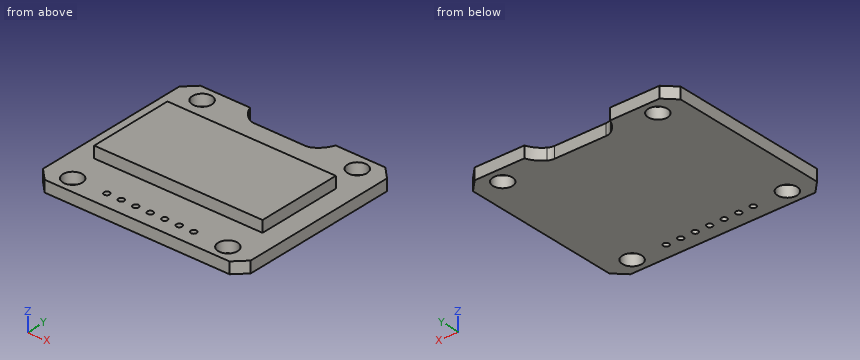
```python
from build123d import *

# Parameters (mm, degrees)
SKETCH_1_W          = 36.4
SKETCH_1_H          = 31.9
EXTRUDE_1_DEPTH     = 2
SKETCH_2_W          = 29.5
SKETCH_2_H          = 15
EXTRUDE_2_DEPTH     = 2
SKETCH_3_R          = 1.7
CUT_EXTRUDE_2_DEPTH = 2
CUT_EXTRUDE_3_DEPTH = 2
SKETCH_5_R          = 0.5
CUT_EXTRUDE_4_DEPTH = 30
CUT_EXTRUDE_5_DEPTH = 10
FILLET_1_R          = 2


with BuildPart() as part:
    # 草图1 → 凸台-拉伸1 (new body)
    with BuildSketch(Plane.XY):
        Rectangle(SKETCH_1_W, SKETCH_1_H)
    extrude(amount=EXTRUDE_1_DEPTH)

    # 草图2 → 凸台-拉伸2 (add)
    with BuildSketch(Plane.XY.offset(2)):
        Rectangle(SKETCH_2_W, SKETCH_2_H)
    extrude(amount=EXTRUDE_2_DEPTH)

    # 草图3 → 切除-拉伸2 (cut)
    with BuildSketch(Plane.XY.offset(2)):
        with Locations((-13.6, 13.25)):
            Circle(SKETCH_3_R)
        with Locations(Location((13.6, 13.25, 0), (0, 0, 180))):
            Circle(SKETCH_3_R)
        with Locations((13.6, -13.25)):
            Circle(SKETCH_3_R)
        with Locations(Location((-13.6, -13.25, 0), (0, 0, 180))):
            Circle(SKETCH_3_R)
    extrude(amount=-CUT_EXTRUDE_2_DEPTH, mode=Mode.SUBTRACT)

    # 草图4 → 切除-拉伸3 (cut)
    with BuildSketch(Plane.XY.offset(2)):
        Polygon((-16.2, 15.95), (-18.2, 13.95), (-18.2, 15.95), align=None)
        Polygon((18.2, 13.95), (18.2, 15.95), (16.2, 15.95), align=None)
        Polygon((16.2, -15.95), (18.2, -13.95), (18.2, -15.95), align=None)
        Polygon((-18.2, -13.95), (-18.2, -15.95), (-16.2, -15.95), align=None)
    extrude(amount=-CUT_EXTRUDE_3_DEPTH, mode=Mode.SUBTRACT)

    # 草图5 → 切除-拉伸4 (cut)
    with BuildSketch(Plane.XY.offset(2)):
        with Locations((-7.62, -13.25)):
            Circle(SKETCH_5_R)
        with Locations((-5.08, -13.25)):
            Circle(SKETCH_5_R)
        with Locations((-2.54, -13.25)):
            Circle(SKETCH_5_R)
        with Locations((0, -13.25)):
            Circle(SKETCH_5_R)
        with Locations((2.54, -13.25)):
            Circle(SKETCH_5_R)
        with Locations((5.08, -13.25)):
            Circle(SKETCH_5_R)
        with Locations((7.62, -13.25)):
            Circle(SKETCH_5_R)
    extrude(amount=-CUT_EXTRUDE_4_DEPTH, mode=Mode.SUBTRACT)

    # 草图6 → 切除-拉伸5 (cut)
    with BuildSketch(Plane.XY.offset(2)):
        with BuildLine():
            Line((-5, 13.25), (5, 13.25))
            ThreePointArc((5, 13.25), (6.519232871, 14.350710305), (7.5, 15.95))
            Line((7.5, 15.95), (-7.5, 15.95))
            ThreePointArc((-7.5, 15.95), (-6.519232871, 14.350710305), (-5, 13.25))
        make_face()
    extrude(amount=-CUT_EXTRUDE_5_DEPTH, mode=Mode.SUBTRACT)

    # 圆角1
    fillet_1_edges = [part.edges().sort_by_distance(p)[0] for p in [
        (-5, 13.25, 1),
        (5, 13.25, 1),
    ]]
    fillet(fillet_1_edges, radius=FILLET_1_R)


solid = part.part
```
Read the model definition and answer for the solid it produces. Units are mm, in the model's axes. Give positions to 0.01 mm unless a question says otherwise; leave off trailing zeros. Write each loop counter-clockwise with the first axis right and the second up, starting at its lowest first coordinate (ties: lowest second). Pieces come first, ordered by that corner, then holes. Notation, with made-up numbers: (83, 65) - (141, 65) arc R29 cw to (141, 95) - close; hole circle Ø4 at (6, -8.75). An arc over 180 degrees is marked (long way). Write item = value, one per line. Start each with the question number.
Item 1: Find section B-B (z = 1.35). State how many separate pieces and enclosed holes the cut face has, then the cut area to 3 significant figures.
Item 2: Find section A-A (x = 2.54). Give the vertices of the cut face in (y, z), then the cut area to 3 significant figures.
Item 3: Find the intervals of material crossed by probe 1 along Y at (x, z) = (13.6, 0.9); probe 2 along Y at (x, z) = (0, 0.2); probe 3 along X at (y, z) = (5, 2.1), in increasing order. Write a range as [from, to].
Item 4: Each of these flat-tipped pins is pushed along its axis until it touches: P1, Ø2, axis at x = 0, z = 2.5, coming from the +Y side; P2, Ø3, axis at x = 13.6, y = 13.25, coming from the -Z side; P3, Ø1.6, axis at y = 3, z = 3, coming from the -X side; P4, Ø1, axis at x = 12.5, z = 3.5, coming from the -Y side. Where does it stop, or does it pass through?
Item 5: Find section C-C (x = -13.6). Give the vertices of the cut face in (y, z), then the cut area to 3 significant figures.
Response:
q1.separate_pieces = 1
q1.enclosed_holes = 11
q1.area = 1,080 mm²
q2.outline = (-15.95, 0) - (-13.75, 0) - (-13.75, 2) - (-15.95, 2) - close; (-12.75, 0) - (13.25, 0) - (13.25, 2) - (7.5, 2) - (7.5, 4) - (-7.5, 4) - (-7.5, 2) - (-12.75, 2) - close
q2.area = 86.4 mm²
q3.probe_1 = [-15.95, -14.95], [-11.55, 11.55], [14.95, 15.95]
q3.probe_2 = [-15.95, -13.75], [-12.75, 13.25]
q3.probe_3 = [-14.75, 14.75]
q4.P1 = 13.25
q4.P2 = through
q4.P3 = -14.75
q4.P4 = -7.5
q5.outline = (-15.95, 0) - (-14.95, 0) - (-14.95, 2) - (-15.95, 2) - close; (-11.55, 0) - (11.55, 0) - (11.55, 2) - (7.5, 2) - (7.5, 4) - (-7.5, 4) - (-7.5, 2) - (-11.55, 2) - close; (14.95, 0) - (15.95, 0) - (15.95, 2) - (14.95, 2) - close
q5.area = 80.2 mm²
